from build123d import *

# Parameters (mm, degrees)
SKIZZE1_R                       = 5.9
AUFSATZ_LINEAR_AUSTRAGEN1_DEPTH = 4
SKIZZE2_R                       = 2.45
SCHNITT_LINEAR_AUSTRAGEN1_DEPTH = 4
SKIZZE3_R                       = 6.915910243
SCHNITT_LINEAR_AUSTRAGEN3_DEPTH = 6


with BuildPart() as part:
    # Skizze1 → Aufsatz-Linear austragen1 (new body)
    with BuildSketch(Plane.XY):
        Circle(SKIZZE1_R)
    extrude(amount=AUFSATZ_LINEAR_AUSTRAGEN1_DEPTH)

    # Skizze2 → Schnitt-Linear austragen1 (cut)
    with BuildSketch(Plane(origin=(0, 0, 0), x_dir=(-1, 0, 0), z_dir=(0, 0, -1))):
        Circle(SKIZZE2_R)
    extrude(amount=-SCHNITT_LINEAR_AUSTRAGEN1_DEPTH, mode=Mode.SUBTRACT)

    # Skizze3 → Schnitt-Linear austragen3 (cut)
    with BuildSketch(Plane(origin=(0, 0, 0), x_dir=(-1, 0, 0), z_dir=(0, 0, -1))):
        Circle(SKIZZE3_R)
        Polygon((0, 5.9), (0.831052654, 4.713133809), (2.017918846, 5.544186463), (2.392920747, 4.144660313), (3.792446897, 4.519662214), (3.666167283, 3.076279615), (5.109549882, 2.95), (4.497219937, 1.636854194), (5.810365743, 1.024524248), (4.785841495, 0), (5.810365743, -1.024524248), (4.497219937, -1.636854194), (5.109549882, -2.95), (3.666167283, -3.076279615), (3.792446897, -4.519662214), (2.392920747, -4.144660313), (2.017918846, -5.544186463), (0.831052654, -4.713133809), (0, -5.9), (-0.831052654, -4.713133809), (-2.017918846, -5.544186463), (-2.392920747, -4.144660313), (-3.792446897, -4.519662214), (-3.666167283, -3.076279615), (-5.109549882, -2.95), (-4.497219937, -1.636854194), (-5.810365743, -1.024524248), (-4.785841495, 0), (-5.810365743, 1.024524248), (-4.497219937, 1.636854194), (-5.109549882, 2.95), (-3.666167283, 3.076279615), (-3.792446897, 4.519662214), (-2.392920747, 4.144660313), (-2.017918846, 5.544186463), (-0.831052654, 4.713133809), align=None, mode=Mode.SUBTRACT)
    extrude(amount=-SCHNITT_LINEAR_AUSTRAGEN3_DEPTH, mode=Mode.SUBTRACT)


solid = part.part
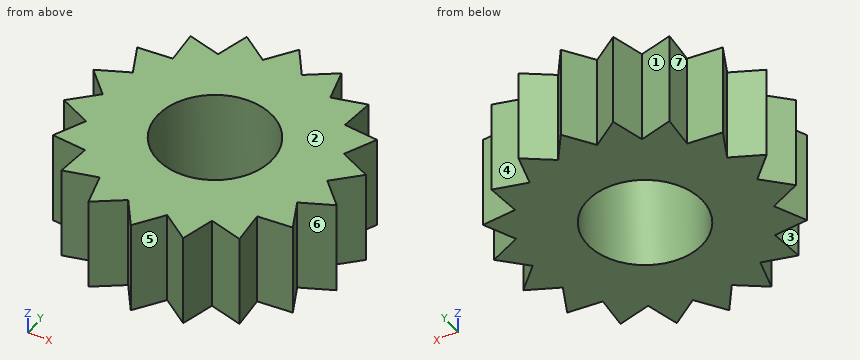
The model under review builds one solid part; all positions refer to its coordinate system, in mm. Face numbers are marked on the shaded views. A direction names the side the tool comes from. Give positions to 0.01 mm unless a question says otherwise; leave off trailing zeros. Loops run counter-clockwise (first coordinate to the right, second up) from the corner with the lowest first, then second, coordinate; pieces in that order, holes last. Notation, with made-up numbers: (70.5, 22) -> (116.5, 22) arc R16 ccw to (116.5, 28) -> close; hole circle Ø3 at (61, 25). An arc over 180 degrees is marked (long way). Put each result on its own line as item: value. Start each with the question number.
1. We need section D-D on x = -3. State the section outline as (y, z) points.
2. We need section C-C on y = 2.75. State the section outline as (x, z) points, then the cut area to 3 significant figures.
3. For the marked faces 4, 5, 6 and 7, list the 3-axis set-ups (+Z, -Z, +X, -X, +Y, -Y) from which the entire face can be reached by the end or side of a thin tool; tool diameter is ignored.
4. Wall thickness on probe 1 along X at (y, z) = (-5, 1.5); probe 2 along Y at (x, z) = (4.75, 0.25); probe 3 along Y at (x, z) = (1.75, 0.6): over which ranges is each line inside the solid? List them lowest first.
5. We need section B-B on y = 5. State the section outline as (x, z) points, then the cut area to 3 significant figures.
6. Clearance check with flat-ended pins moving along their axes: P1, Ø1, axis at y = 4.5, z = 2.5, coming from the -X side; P2, Ø1.5, axis at y = 3.5, z = 2.5, coming from the +X side. State where each tip first meets the part, or that it passes through.
7. We need section A-A on x = -1.75. State the section outline as (y, z) points.
8. Mouldability with a two-part tool opening along X and no side actions: class the marked faces 1, 2 and 3 as released by +X, released by -X, zero draft, split by the parting line, or undercut.
Determined:
1. outline: (-4.31, 0) -> (4.31, 0) -> (4.31, 4) -> (-4.31, 4) -> close
2. outline: (-5.02, 0) -> (5.02, 0) -> (5.02, 4) -> (-5.02, 4) -> close
2. area: 40.1 mm^2
3. face 4: +Z, -Z, +Y
3. face 5: +Z, -Z, -Y
3. face 6: +Z, -Z, +X
3. face 7: +Z, -Z, -X
4. probe 1: -2.16 to -1.24, -0.63 to 0.63, 1.24 to 2.16
4. probe 2: -2.98 to -2.18, -1.52 to 1.52, 2.18 to 2.98
4. probe 3: -5.36 to -1.71, 1.71 to 5.36
5. outline: (-2.16, 0) -> (-1.24, 0) -> (-1.24, 4) -> (-2.16, 4) -> close; (-0.63, 0) -> (0.63, 0) -> (0.63, 4) -> (-0.63, 4) -> close; (1.24, 0) -> (2.16, 0) -> (2.16, 4) -> (1.24, 4) -> close
5. area: 12.4 mm^2
6. P1: x = -3.79
6. P2: x = 5.11
7. outline: (-5.36, 0) -> (-1.71, 0) -> (-1.71, 4) -> (-5.36, 4) -> close; (1.71, 0) -> (5.36, 0) -> (5.36, 4) -> (1.71, 4) -> close
8. face 1: undercut
8. face 2: zero draft
8. face 3: released by -X
